from build123d import *

# Parameters (mm, degrees)
F1_DEPTH  = 38.1
F2_W      = 71.12
F2_H      = 27.3908400369
F3_DEPTH  = 50.8
F4_W      = 25.4
F4_H      = 19.05
F5_DEPTH  = 228.6
F7_DEPTH  = 6.35
F8_W      = 12.7
F8_H      = 165.1
F9_DEPTH  = 6.35
F10_W     = 6.35
F10_H     = 161.925
F11_DEPTH = 127
F13_DEPTH = 6.35
F14_W     = 12.7
F14_H     = 15.3125979424
F15_DEPTH = 6.35
F16_R     = 8.1334843178
F17_DEPTH = 76.2
F18_R     = 5.08
F20_DEPTH = 76.2


with BuildPart() as f1:
    # F0 (on Front) → F1 (new body, symmetric)
    with BuildSketch(Plane.XZ):
        Polygon((30.48, -22.225), (49.53, -22.225), (49.53, 22.225), (-49.53, 22.225), (-49.53, -22.225), (-30.48, -22.225), (-30.48, 3.175), (30.48, 3.175), align=None)
    extrude(amount=F1_DEPTH, both=True)

    # F2 (on Front) → F3 (cut, symmetric)
    with BuildSketch(Plane.XZ):
        with Locations((0, -23.2204200185)):
            Rectangle(F2_W, F2_H)
    extrude(amount=F3_DEPTH, both=True, mode=Mode.SUBTRACT)

    # F4 (on face) → F5 (join)
    with BuildSketch(Plane.XY.offset(22.225)):
        with Locations((-36.83, -28.575)):
            Rectangle(F4_W, F4_H)
    extrude(amount=F5_DEPTH)

    # F6 (on face) → F7 (join)
    with BuildSketch(Plane.XZ.offset(38.1)):
        Polygon((-24.13, 73.025), (-24.13, 22.225), (13.97, 22.225), align=None)
    extrude(amount=-F7_DEPTH)

    # F8 (on face) → F9 (cut)
    with BuildSketch(Plane(origin=(0, -19.05, 0), x_dir=(-1, 0, 0), z_dir=(0, 1, 0))):
        with Locations((36.83, 161.925)):
            Rectangle(F8_W, F8_H)
    extrude(amount=-F9_DEPTH, mode=Mode.SUBTRACT)

    # F10 (on Front) → F11 (cut)
    with BuildSketch(Plane.XZ):
        with Locations((-36.83, 160.3375)):
            Rectangle(F10_W, F10_H)
    extrude(amount=F11_DEPTH, mode=Mode.SUBTRACT)

    # F12 (on face) → F13 (join)
    with BuildSketch(Plane(origin=(-49.53, 0, 0), x_dir=(0, -1, 0), z_dir=(-1, 0, 0))):
        Polygon((-19.05, 22.225), (19.05, 22.225), (19.05, 73.025), align=None)
    extrude(amount=-F13_DEPTH)

    # F14 (on face) → F15 (cut)
    with BuildSketch(Plane(origin=(0, -19.05, 0), x_dir=(-1, 0, 0), z_dir=(0, 1, 0))):
        with Locations((36.83, 244.475)):
            Rectangle(F14_W, F14_H)
    extrude(amount=-F15_DEPTH, mode=Mode.SUBTRACT)

    # F16 (on face) → F17 (join)
    with BuildSketch(Plane.XZ.offset(38.1)):
        with Locations((-35.56, -9.525)):
            Circle(F16_R)
    extrude(amount=-F17_DEPTH)

    # F18
    f18_edges = [f1.edges().sort_by_distance(p)[0] for p in [
        (-35.56, 0, -17.658484),
    ]]
    fillet(f18_edges, radius=F18_R)

    # F19 (on face) → F20 (join)
    with BuildSketch(Plane.XZ.offset(38.1)):
        Polygon((35.56, -9.525), (30.48, -9.525), (35.56, -15.875), align=None)
    extrude(amount=-F20_DEPTH)


solid = f1.part
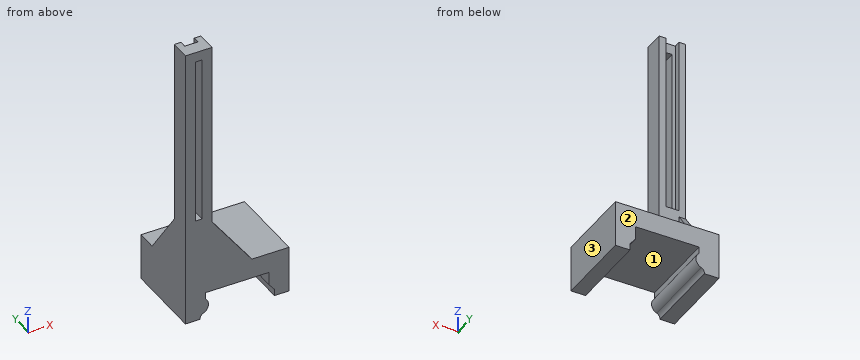
The listing builds one solid part. Answer for the finished solid, in the listing's coordinates (mm). Face numbers are marked on the shaded views. Give positions to 0.01 mm unless a question says otherwise; leave off trailing zeros. Order: outer loops, then holes, each group sorted by start corner. A loop starts at its lowest first (then second) coordinate and runs counter-clockwise, first axis right, second up. Notation, with made-up numbers: (-11, 80) - (-6, 80) arc R18 ccw to (-6, 114) - close; hole circle Ø6 at (40, 79.25). An arc over 180 degrees is marked (long way). Use one line per item in the form item = value.
1) The mould has two halves that part along X. Classify the marked faces 1, 2 and 3: released by +X, released by -X, zero draft, split by the parting line, or undercut.
Verdict:
face_1 = undercut
face_2 = zero draft
face_3 = released by +X
2) Find section A-A on z = 202. Determine the outline of the cut face in (x, y) (3 decimals).
Verdict:
outline = (-49.53, -38.1) - (-40.005, -38.1) - (-40.005, -25.4) - (-43.18, -25.4) - (-43.18, -19.05) - (-49.53, -19.05) - close; (-33.655, -38.1) - (-24.13, -38.1) - (-24.13, -19.05) - (-30.48, -19.05) - (-30.48, -25.4) - (-33.655, -25.4) - close
3) Each of these flat-tipped pins is pushed along its axis until it touches: pin 1 (21 mm diameter, centred on y = -27.5, z = 172, fed in from +X); pin 2 (11.5 mm diameter, centred on x = -14, z = 42, fed in from +Y); pin 3 (12.5 mm diameter, centred on x = -33.5, z = 172.5, fed in from +Y). Where does it stop, or does it pass through?
Verdict:
pin_1 = -24.13
pin_2 = -31.75
pin_3 = -19.05
4) Consider probe 1 along X at (y, z) = (-33.5, 106) (3 decimals); probe 2 along Y at (x, z) = (-44, 214.5); probe 3 along X at (y, z) = (-20, 160). Determine where each line is inside the solid, lowest interval first. Write a range as [from, to].
Verdict:
probe_1 = [-49.53, -40.005], [-33.655, -24.13]
probe_2 = [-38.1, -19.05]
probe_3 = [-49.53, -43.18], [-30.48, -24.13]
5) Find section C-C on z = 37.5. Determine the outline of the cut face in (x, y).
Verdict:
outline = (-49.53, -38.1) - (2.51, -38.1) - (2.51, -31.75) - (-24.13, -31.75) - (-24.13, -19.05) - (-43.18, -19.05) - (-43.18, 7.59) - (-49.53, 7.59) - close
6) Find section B-B on y = 22. Determine the outline of the cut face in (x, z) (3 decimals), and give its area (3 significant figures).
Verdict:
outline = (-49.53, -22.225) - (-35.56, -22.225) - (-35.56, -21.723) arc R5.08 cw to (-32.433, -17.033) arc R8.133 ccw to (-30.48, -3.173) - (-30.48, 3.175) - (30.48, 3.175) - (30.48, -9.525) - (35.56, -15.875) - (35.56, -22.225) - (49.53, -22.225) - (49.53, 22.225) - (-49.53, 22.225) - close
area = 2,810 mm^2
7) Find section D-D on x = -4. Determine the outline of the cut face in (y, z) (3 decimals).
Verdict:
outline = (-38.1, 3.175) - (38.1, 3.175) - (38.1, 22.225) - (-31.75, 22.225) - (-31.75, 46.185) - (-38.1, 46.185) - close
